Work out the finished part from the listing and answer in its coordinate system (mm). A direction names the side the tool comes from. Round coordinates to 2 decimals unless told otherwise and drop trailing zeros. Loops run counter-clockwise (first coordinate to the right, second up) from the corner with the lowest first, then second, coordinate; pieces in that order, holes last. Notation, with made-up numbers: M 62,70.25 L 110,70.25 A11 cw 110,83.25 Z; hole C -31,1.25 d2. An arc over 180 degrees is marked long. One line per item, written item: value.
```python
from build123d import *

# Parameters (mm, degrees)
F0_W     = 192
F0_H     = 8
F0_W_2   = 8
F0_H_2   = 192
F1_DEPTH = 100
F2_R     = 7.5
F3_DEPTH = 8
F4_R     = 7.5
F5_DEPTH = 8


with BuildPart() as f1:
    # F0 (on Top) → F1 (new body)
    with BuildSketch(Plane.XY):
        with Locations((0.652894, 118.005262)):
            Rectangle(F0_W, F0_H)
        with Locations((-99.347106, 118.005262)):
            Rectangle(F0_W_2, F0_H)
        with Locations((-99.347106, 18.005262)):
            Rectangle(F0_W_2, F0_H_2)
    extrude(amount=F1_DEPTH)

    # F2 (on face) → F3 (cut)
    with BuildSketch(Plane.XZ.offset(-114.005262)):
        with Locations((-53.347106, 50)):
            Circle(F2_R)
        with Locations((46.652894, 50)):
            Circle(F2_R)
    extrude(amount=-F3_DEPTH, mode=Mode.SUBTRACT)

    # F4 (on face) → F5 (cut)
    with BuildSketch(Plane.YZ.offset(-95.347106)):
        with Locations((-27.994738, 50)):
            Circle(F4_R)
        with Locations((72.005262, 50)):
            Circle(F4_R)
    extrude(amount=-F5_DEPTH, mode=Mode.SUBTRACT)


solid = f1.part
```
1) Find section C-C (z = 73). Give the vertices of the cut face in (x, y), then the cut area to 3 significant figures.
Check values:
outline: M -103.35,-77.99 L -95.35,-77.99 L -95.35,114.01 L 96.65,114.01 L 96.65,122.01 L -103.35,122.01 Z
area: 3,140 mm2
2) Find section B-B (y = 76). Give the vertices of the cut face in (x, z).
Check values:
outline: M -103.35,0 L -95.35,0 L -95.35,43.65 L -103.35,43.65 Z; M -103.35,56.35 L -95.35,56.35 L -95.35,100 L -103.35,100 Z
3) The mould has two halves that part along X. Classify faces 3 (the face through (-99, -77.995, 49)), 4 (the face through (-103.347, 23, 49)), 5 (the face through (-49.886, 117.949, 43.346)): +X half, -X half, draft (parallel to the pull), parting line (faces both ways), or undercut.
Check values:
face 3: draft
face 4: -X half
face 5: undercut
4) Find section D-D (x = 24). Give the vertices of the cut face in (y, z), then the cut area to 3 significant figures.
Check values:
outline: M 114.01,0 L 122.01,0 L 122.01,100 L 114.01,100 Z
area: 800 mm2
5) For faces 1 (the face through (50.114, 117.949, 43.346)), 2 (the face through (-95.347, 17, 49)), determine the directions among +Z, -Z, +X, -X, +Y, -Y from which every point of the face is accessible in a straight line to the end or side of a thin tool.
Check values:
face 1: +Y, -Y
face 2: +Z, -Z, +X, -Y
6) Find section A-A (z = 50). Give the vertices of the cut face in (x, y), then the cut area to 3 significant figures.
Check values:
outline: M -103.35,-77.99 L -95.35,-77.99 L -95.35,-35.49 L -103.35,-35.49 Z; M -103.35,-20.49 L -95.35,-20.49 L -95.35,64.51 L -103.35,64.51 Z; M -103.35,79.51 L -95.35,79.51 L -95.35,114.01 L -60.85,114.01 L -60.85,122.01 L -103.35,122.01 Z; M -45.85,114.01 L 39.15,114.01 L 39.15,122.01 L -45.85,122.01 Z; M 54.15,114.01 L 96.65,114.01 L 96.65,122.01 L 54.15,122.01 Z
area: 2,660 mm2
7) Each of these flat-tipped pins is pushed along its axis until it touches: pin 1 (2 mm diameter, centred on x = -21.5, z = 79.5, fed in from -Y); pin 2 (6 mm diameter, centred on y = -14.5, z = 60, fed in from +X). Where does it stop, or does it pass through?
Check values:
pin 1: y = 114.01
pin 2: x = -95.35
8) Find the intervals of material crossed by probe 1 along Y at (x, z) = (-37, 9.5); probe 2 along X at (y, z) = (73.5, 7), in increasing order. Write a range as from..to.
Check values:
probe 1: 114.01..122.01
probe 2: -103.35..-95.35
